For this review, take the finished solid that the model builds, in its own axes (mm). A direction names the side the tool comes from. Coordinates: 2 decimals unless noted, no trailing zeros. Write each loop counter-clockwise with the first axis right and the second up, starting at its lowest first coordinate (ties: lowest second). Pieces come first, ordered by that corner, then holes. Notation, with made-up numbers: M 66.5,88.25 L 116.5,88.25 A34 ccw 116.5,120.25 Z; hole C -14,75.5 d6. An arc over 180 degrees is marked long. One line per question, with ' | ' between items.
from build123d import *

# Parameters (mm, degrees)
F1_DEPTH = 586.74
F2_DEPTH = 586.74


with BuildPart() as f1:
    # F0 (on Front) → F1 (new body)
    with BuildSketch(Plane.XZ):
        Polygon((-15.55056, -26.781248), (-15.55056, 24.018752), (-21.90056, 24.018752), (-21.90056, -33.131248), (35.24944, -33.131248), (35.24944, -26.781248), align=None)
    extrude(amount=F1_DEPTH)

    # F1_face (on face) → F2 (join)
    with BuildSketch(Plane(origin=(-5.278502, 0, -16.509189), x_dir=(1, 0, 0), z_dir=(0, 1, 0))):
        Polygon((-10.272059, -40.527941), (-10.272059, 10.272059), (40.527941, 10.272059), (40.527941, 16.622059), (-16.622059, 16.622059), (-16.622059, -40.527941), align=None)
    extrude(amount=F2_DEPTH)


solid = f1.part
1) To check wall thickness, follow line 1 along X through (y, z) = (123, -0.5); line 2 along Z through (x, y) = (-3.5, 445). State the ranges of each line that lie inside material, in increasing order. Write a range as [from, to].
Responses:
line 1: [-21.9, -15.55] | line 2: [-33.13, -26.78]
2) Machinability: for faces 1 (the flat face through (-17, 586.74, -17)), 2 (the flat face through (-15.551, -289, -2)), which of the approach directions +Z, -Z, +X, -X, +Y, -Y give a long, thin tool a straight path to every point of the face, cutting with its end or side? Answer none if there is none.
Responses:
face 1: +Z, -Z, +X, -X, +Y | face 2: +Z, +X, +Y, -Y
3) We need section C-C on x = 19. State the section outline as (y, z) points, then the cut area to 3 significant figures.
Responses:
outline: M -586.74,-33.13 L 586.74,-33.13 L 586.74,-26.78 L -586.74,-26.78 Z | area: 7,450 mm^2
4) Insertion check: pin 1 Ø5 at (y, z) = (-314, -13.5) entering from +X; pin 2 Ø12 at (x, z) = (17, -20.5) entering from +Y; pin 3 Ø2 at (x, y) = (10.5, -394.5) entering from +Z. Each pin has a flat end and moves straight along its axis. Give the tip position at first contact, or say it passes through.
Responses:
pin 1: x = -15.55 | pin 2: through | pin 3: z = -26.78
5) We need section B-B on y = -480.5. State the section outline as (x, z) points, then the cut area to 3 significant figures.
Responses:
outline: M -21.9,-33.13 L 35.25,-33.13 L 35.25,-26.78 L -15.55,-26.78 L -15.55,24.02 L -21.9,24.02 Z | area: 685 mm^2
